The drawing under review shows one solid part. Ordinate dimensions are in mm from its lowest x, y, z. Round coordinates to 2 decimals unless told otherwise and drop trailing zeros. Order: outer loops, then holes, each group sorted by start corner. A loop starts at its lowest first (then second) coordinate and runs counter-clockwise, first axis right, second up. Notation, with made-up numbers: M 21.25,50 L 54.25,50 A34 ccw 54.25,82 Z; hole C 63.25,69.25 d4. An arc over 180 degrees is marked long. Answer as a JSON object with one key per item and string values. Group by question number.
1) The part is to be moulded in two halves that separate along Z. For the marked faces 1 and 2, say which applies: +Z half, -Z half, draft (parallel to the pull), parting line (faces both ways), or undercut.
2) To check wall thickness, follow line 1 (Y direction, x = 1.75, z = 6.25); line 2 (X direction, y = 5.5, z = 7.5); line 3 (Z direction, x = 1.25, y = 9.25). State the ranges of each line that lie inside material, in increasing order.
3) Consider section C-C, the plane x = 1.7. Write out the cut boundary in (y, z), then the cut area to 3 significant figures.
4) Consider section D-D, the plane y = 1.75. Write out the cut boundary in (x, z).
5) Consider section A-A, the plane z = 3.75. Write out the cut boundary in (x, y), then the cut area to 3 significant figures.
6) Insertion check: pin 1 Ø2.5 at (y, z) = (5, 3.5) entering from +X. The pin has a flat end and moves straight along its axis. Give the tip position at first contact, or say it passes through.
7) Consider section B-B, the plane y = 9.25. Write out the cut boundary in (x, z), then the cut area to 3 significant figures.
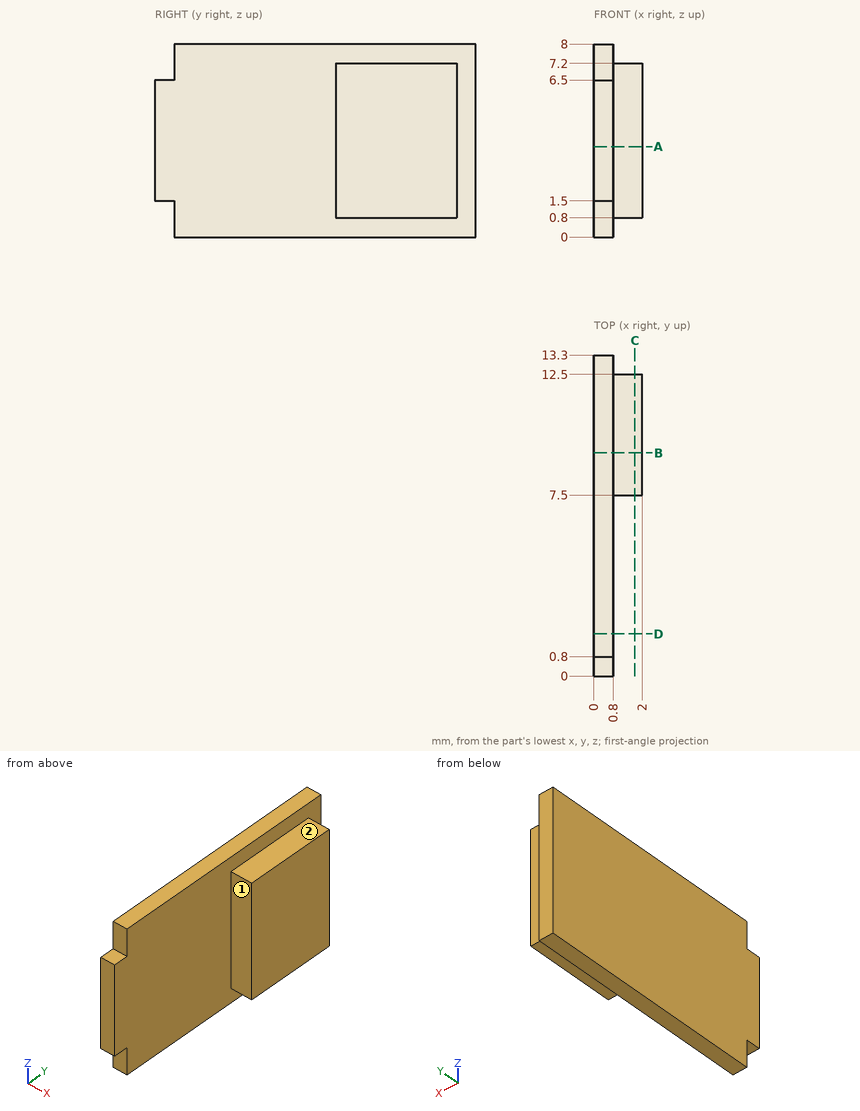
Results list:
{
 "1": {"face 1": "draft", "face 2": "+Z half"},
 "2": {"line 1": "7.5 to 12.5", "line 2": "0 to 0.8", "line 3": "0.8 to 7.2"},
 "3": {"outline": "M 7.5,0.8 L 12.5,0.8 L 12.5,7.2 L 7.5,7.2 Z", "area": "32.0 mm^2"},
 "4": {"outline": "M 0,0 L 0.8,0 L 0.8,8 L 0,8 Z"},
 "5": {"outline": "M 0,0 L 0.8,0 L 0.8,7.5 L 2,7.5 L 2,12.5 L 0.8,12.5 L 0.8,13.3 L 0,13.3 Z", "area": "16.6 mm^2"},
 "6": {"pin 1": "x = 0.8"},
 "7": {"outline": "M 0,0 L 0.8,0 L 0.8,0.8 L 2,0.8 L 2,7.2 L 0.8,7.2 L 0.8,8 L 0,8 Z", "area": "14.1 mm^2"}
}
